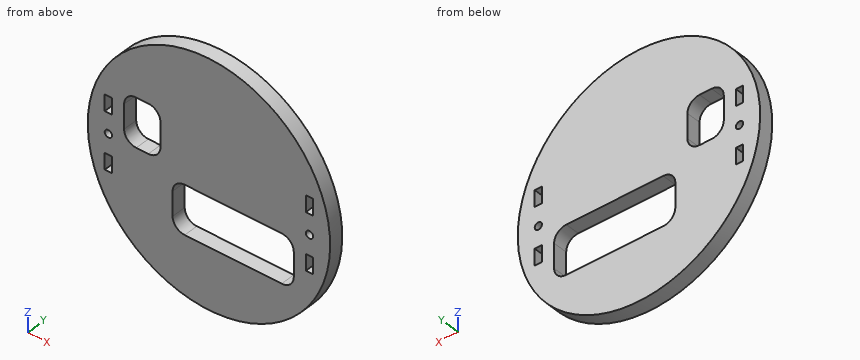
```python
from build123d import *

# Parameters (mm, degrees)
SKETCH2_R           = 50
SKETCH2_R_2         = 1.5
SKETCH2_W           = 3
SKETCH2_H           = 6.7
BOSS_EXTRUDE2_DEPTH = 6


with BuildPart() as part:
    # Sketch2 → Boss-Extrude2 (new body)
    with BuildSketch(Plane(origin=(0, 0, 0), x_dir=(1, 0, 0), z_dir=(0, 1, 0))):
        with Locations(Location((-8.417247628, 8.35921329, 0), (0, 0, 270))):
            Circle(SKETCH2_R)
        with Locations(Location((33.082752372, 8.35921329, 0), (0, 0, 270))):
            Circle(SKETCH2_R_2, mode=Mode.SUBTRACT)
        with Locations(Location((-49.917247628, 8.35921329, 0), (0, 0, 270))):
            Circle(SKETCH2_R_2, mode=Mode.SUBTRACT)
        with Locations((-49.917247628, 20.00921329)):
            Rectangle(SKETCH2_W, SKETCH2_H, mode=Mode.SUBTRACT)
        with Locations((-49.917247628, -3.29078671)):
            Rectangle(SKETCH2_W, SKETCH2_H, mode=Mode.SUBTRACT)
        with Locations((33.082752372, 20.00921329)):
            Rectangle(SKETCH2_W, SKETCH2_H, mode=Mode.SUBTRACT)
        with Locations((33.082752372, -3.29078671)):
            Rectangle(SKETCH2_W, SKETCH2_H, mode=Mode.SUBTRACT)
        with BuildLine():
            Line((21.582752372, 33.35921329), (-18.417247628, 33.35921329))
            ThreePointArc((-18.417247628, 33.35921329), (-21.952781534, 31.894747196), (-23.417247628, 28.35921329))
            Line((-23.417247628, 28.35921329), (-23.417247628, 18.35921329))
            ThreePointArc((-23.417247628, 18.35921329), (-21.952781534, 14.823679384), (-18.417247628, 13.35921329))
            Line((-18.417247628, 13.35921329), (21.582752372, 13.35921329))
            ThreePointArc((21.582752372, 13.35921329), (25.118286278, 14.823679384), (26.582752372, 18.35921329))
            Line((26.582752372, 18.35921329), (26.582752372, 28.35921329))
            ThreePointArc((26.582752372, 28.35921329), (25.118286278, 31.894747196), (21.582752372, 33.35921329))
        make_face(mode=Mode.SUBTRACT)
        with BuildLine():
            Line((-33.417247628, 8.35921329), (-38.417247628, 8.35921329))
            ThreePointArc((-38.417247628, 8.35921329), (-41.952781534, 6.894747196), (-43.417247628, 3.35921329))
            Line((-43.417247628, 3.35921329), (-43.417247628, -6.64078671))
            ThreePointArc((-43.417247628, -6.64078671), (-41.952781534, -10.176320616), (-38.417247628, -11.64078671))
            Line((-38.417247628, -11.64078671), (-33.417247628, -11.64078671))
            ThreePointArc((-33.417247628, -11.64078671), (-29.881713722, -10.176320616), (-28.417247628, -6.64078671))
            Line((-28.417247628, -6.64078671), (-28.417247628, 3.35921329))
            ThreePointArc((-28.417247628, 3.35921329), (-29.881713722, 6.894747196), (-33.417247628, 8.35921329))
        make_face(mode=Mode.SUBTRACT)
    extrude(amount=BOSS_EXTRUDE2_DEPTH)


solid = part.part
```
Verification items for the finished model (mm, model axes). Coordinates: 2 decimals unless noted, no trailing zeros. Order: outer loops, then holes, each group sorted by start corner. A loop starts at its lowest first (then second) coordinate and runs counter-clockwise, first axis right, second up. Notation, with made-up numbers: (24, 21) - (42, 21) arc R20 ccw to (42, 31) - close; hole circle Ø4 at (-11, -15.5). An arc over 180 degrees is marked (long way). Return JSON: item names as keys, results as strings.
(1) Go/stop test with flat-tipped pins: pin 1 (3 mm diameter, centred on y = 4, z = -38, fed in from +X); pin 2 (2 mm diameter, centred on x = 27.5, z = 30.5, fed in from +Y); pin 3 (2.5 mm diameter, centred on x = 33, y = 4, fed in from +Z); pin 4 (2.5 mm diameter, centred on x = -49.5, y = 2, fed in from +Z). Record where each tip stops, or that it passes through.
Filled sheet:
{"pin 1": "stops at x = 32.91", "pin 2": "passes through", "pin 3": "stops at z = 21.42", "pin 4": "stops at z = 21.86"}
(2) Section check D-D, the plane x = 16. Record the cut outline in (y, z).
Filled sheet:
{"outline": "(0, -51.99) - (6, -51.99) - (6, -33.36) - (0, -33.36) - close; (0, -13.36) - (6, -13.36) - (6, 35.27) - (0, 35.27) - close"}
(3) Section check C-C, the plane y = 4.6. Give the number of separate pieces and of enclosed holes in the cut face, and give its area (3 significant figures).
Filled sheet:
{"separate pieces": "1", "enclosed holes": "8", "area": "6,500 mm^2"}
(4) Thickness scan on line 1 along Z through (x, y) = (-9, 0.3); line 2 along X through (y, z) = (4.1, -19); line 3 along X through (y, z) = (1.95, -17). Record the ranges inside material, lowest first.
Filled sheet:
{"line 1": "z = -58.36 to -33.36, -13.36 to 41.64", "line 2": "x = -57.27 to -51.42, -48.42 to -23.42, 26.58 to 31.58, 34.58 to 40.44", "line 3": "x = -57.66 to -51.42, -48.42 to -23.23, 26.39 to 31.58, 34.58 to 40.83"}
(5) Section check B-B, the plane z = -21. Record the cut outline in (x, y).
Filled sheet:
{"outline": "(-56.79, 0) - (-51.42, 0) - (-51.42, 6) - (-56.79, 6) - close; (-48.42, 0) - (-23.42, 0) - (-23.42, 6) - (-48.42, 6) - close; (26.58, 0) - (31.58, 0) - (31.58, 6) - (26.58, 6) - close; (34.58, 0) - (39.96, 0) - (39.96, 6) - (34.58, 6) - close"}
(6) Section check A-A, the plane x = 1. Record the cut outline in (y, z), and give its area (3 significant figures).
Filled sheet:
{"outline": "(0, -57.46) - (6, -57.46) - (6, -33.36) - (0, -33.36) - close; (0, -13.36) - (6, -13.36) - (6, 40.75) - (0, 40.75) - close", "area": "469 mm^2"}
